Geometry: final body of the model. Coordinates: model frame, mm. A direction names the side the tool comes from. Give positions to 0.01 mm unless a question says otherwise; leave off trailing zeros. Loops run counter-clockwise (first coordinate to the right, second up) from the corner with the lowest first, then second, coordinate; pieces in that order, holes last.
Autodesk Inventor part; units mm, degrees
ref_plane "YZ Plane" through (0, 0, 0) normal (1, 0, 0) x (0, 1, 0)
ref_plane "XZ Plane" through (0, 0, 0) normal (0, 1, 0) x (-1, 0, 0)
ref_plane "XY Plane" through (0, 0, 0) normal (0, 0, 1) x (1, 0, 0)
sketch "草圖1" plane through (0, 0, 0) normal (0, 1, 0) x (-1, 0, 0)
  line L0 (0, 0) -> (10, 0)
  line L1 (10, 0) -> (10, -10)
  line L2 (10, -10) -> (0, -10)
  line L3 (0, -10) -> (0, 0)
  circle A0 centre (7.5, -2.5) radius 1.7
  circle A1 centre (7.5, -7.5) radius 1.7
  circle A2 centre (2.5, -2.5) radius 1.7
  circle A3 centre (2.5, -7.5) radius 1.7
  dimension "d0" = 10
  dimension "d1" = 10
  dimension "d2" = 3.4
  dimension "d3" = 2.5
  dimension "d4" = 2.5
  dimension "d7" = 5
  dimension "d10" = 5
extrude "擠出1" add sketch "草圖1" against normal blind 5 contours L0 L1 L2 L3 | A0 | A1 | A2 | A3
sketch "草圖1 outline for 擠出2" plane through (0, 0, 0) normal (0, 1, 0) x (-1, 0, 0)
  line L0 (0, 0) -> (0, -10)
  line L1 (10, 0) -> (0, 0)
  line L2 (10, -10) -> (10, 0)
  line L3 (0, -10) -> (10, -10)
extrude "擠出2" add sketch "草圖1 outline for 擠出2" along normal blind 10 draft -30
sketch "草圖2" plane through (0, -5, 0) normal (0, -1, 0) x (1, 0, 0)
  circle A0 centre (-7.5, -7.5) radius 1.7
  line L0 (-10, -10) -> (0, -10)
  line L1 (0, -10) -> (0, 0)
  line L2 (0, 0) -> (-10, 0)
  line L3 (-10, 0) -> (-10, -10)
extrude "擠出3" cut sketch "草圖2" against normal blind 1.5 contours A0
pattern_linear "矩形陣列1" count 2 spacing 5 along (0, 0, 1) count 2 spacing 5 along (1, 0, 0) of "擠出3"
properties part number "110033226_ipt_35_中心城堡圍牆頂部_MIR"
Item 1: Draft query along Z for faces 1 (the face through (-7.87, -4.26, -9.16)), 2 (the face through (0, -2, -5)), 3 (the face through (-4.93, 3.31, -1.91)). Return one class per face: +Z half, -Z half, draft (parallel to the pull), parting line (faces both ways), or undercut.
Values follow:
face 1: undercut
face 2: draft
face 3: +Z half
Item 2: Section query B-B on z = -2.5. Return loops of the section in (x, y), plus the area to 3 significant figures.
Values follow:
outline: (-10, -5) - (-9.2, -5) - (-9.2, -3.5) - (-5.8, -3.5) - (-5.8, -5) - (-4.2, -5) - (-4.2, -3.5) - (-0.8, -3.5) - (-0.8, -5) - (0, -5) - (0, 0) - (-2.5, 4.33) - (-7.5, 4.33) - (-10, 0) - close
area: 72.3 mm2
Item 3: Section query C-C on y = 3.5. Return loops of the section in (x, z), plus the area to 3 significant figures.
Values follow:
outline: (-7.98, -7.98) - (-2.02, -7.98) - (-2.02, -2.02) - (-7.98, -2.02) - close
area: 35.5 mm2
Item 4: Set-up query: faces 4 (the face through (-0.88, -4.26, -1.99)), 5 (the face through (-5, -2, -10)). Return all of +Z, -Z, +X, -X, +Y, -Y with unobstructed straight access to the full face (end or side cutting, diameter ignored); none if empty.
Values follow:
face 4: -Y
face 5: -Z, +X, -X, +Y, -Y
Item 5: Section query A-A on x = -3.5. Return loops of the section in (y, z), plus the area to 3 significant figures.
Values follow:
outline: (-5, -10) - (0, -10) - (6.06, -6.5) - (6.06, -3.5) - (0, 0) - (-5, 0) - (-5, -1.13) - (-3.5, -1.13) - (-3.5, -3.87) - (-5, -3.87) - (-5, -6.13) - (-3.5, -6.13) - (-3.5, -8.87) - (-5, -8.87) - close
area: 81.2 mm2
Item 6: Pin query (flat end, axial travel): pin 1 (1 mm diameter, centred on x = -4, y = 1.5, fed in from +Z); pin 2 (2.5 mm diameter, centred on x = -2.5, z = -7.5, fed in from -Y); pin 3 (3 mm diameter, centred on x = -7.5, z = -7.5, fed in from +Y). Return the tip coordinate at first contact, or that it passes through.
Values follow:
pin 1: stops at z = -0.58
pin 2: stops at y = -3.5
pin 3: stops at y = 6.17
Item 7: Ray query, probe 1 along Z at (x, y) = (-2.5, -4.7); probe 2 along Z at (x, y) = (-7, -3.75); probe 3 along X at (y, z) = (-3.75, -4). Return the intervals inside material, ascending.
Values follow:
probe 1: z = -10 to -9.2, -5.8 to -4.2, -0.8 to 0
probe 2: z = -10 to -9.12, -5.88 to -4.12, -0.88 to 0
probe 3: x = -10 to -8.3, -6.7 to -3.3, -1.7 to 0
